The figure shows three views and two pictorial views of one solid part (mm, origin at its lowest corner). Answer the questions. Coordinates: 2 decimals unless noted, no trailing zeros. Order: outer loops, then holes, each group sorted by start corner. A loop starts at its lowest first (then second) coordinate and runs counter-clockwise, first axis right, second up.
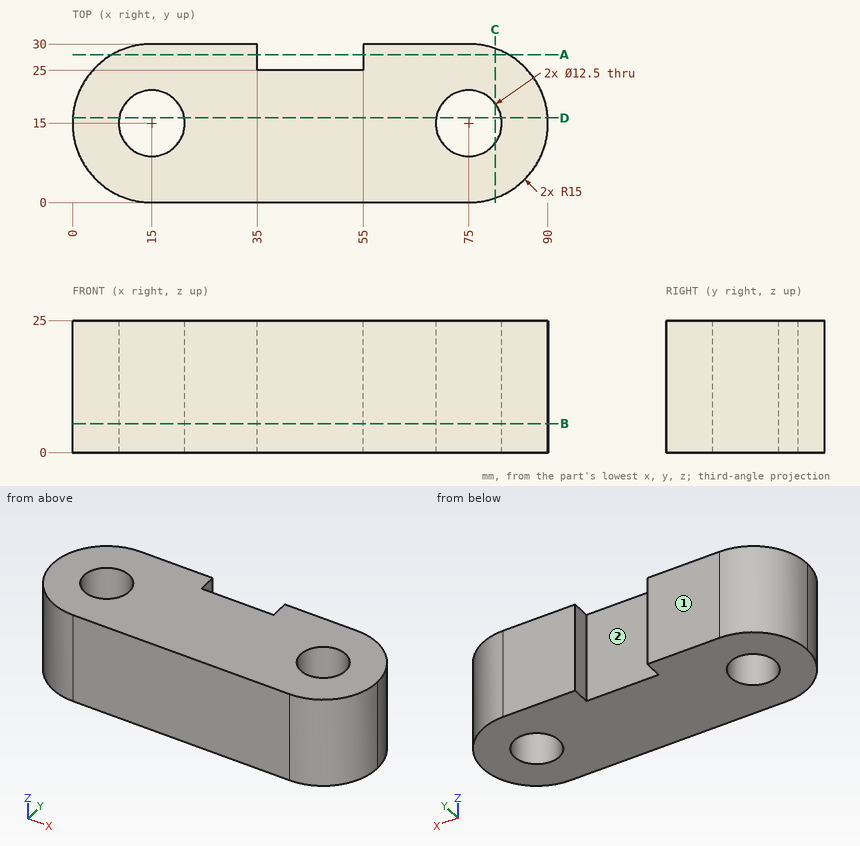
Q1. Determine the mould class of the marked faces 1 and 2 for opening direction X: +X half, -X half, draft (parallel to the pull), parting line (faces both ways), or undercut.
Q2. The part is cut by section B-B, the plane z = 5.5. Determine the outline of the cut face in (x, y).
Q3. The part is cut by section C-C, the plane x = 80. Determine the outline of the cut face in (y, z).
Q4. Each of these flat-tipped pins is pushed along its axis until it touches: P1, Ø11, axis at x = 75, y = 15, coming from the +Z side; P2, Ø3, axis at x = 44, y = 7.5, coming from the -Z side; P3, Ø5.5, axis at y = 28, z = 16.5, coming from the -X side; P4, Ø1.5, axis at y = 22, z = 16.5, coming from the -X side. Where does it stop, or does it pass through?
Q5. The part is cut by section A-A, the plane y = 28. Determine the outline of the cut face in (x, z).
Q6. The part is cut by section D-D, the plane y = 16. Determine the outline of the cut face in (x, z).
Q7. Straight lines are drawn through the part: L1, parallel to X at y = 16, z = 21.5; L2, parallel to X at y = 17, z = 24.25; L3, parallel to Y at x = 16.5, z = 23.5. For each, find the intervals that lie inside material, in ascending order.
Computed values:
1. face 1: draft
1. face 2: undercut
2. outline: (0, 15) arc R15 ccw to (15, 0) - (75, 0) arc R15 ccw to (90, 15) arc R15 ccw to (75, 30) - (55, 30) - (55, 25) - (35, 25) - (35, 30) - (15, 30) arc R15 ccw to start; hole circle Ø12.5 at (15, 15); hole circle Ø12.5 at (75, 15)
3. outline: (0.86, 0) - (11.25, 0) - (11.25, 25) - (0.86, 25) - close; (18.75, 0) - (29.14, 0) - (29.14, 25) - (18.75, 25) - close
4. P1: passes through
4. P2: stops at z = 0
4. P3: stops at x = 4.05
4. P4: stops at x = 1.36
5. outline: (7.52, 0) - (35, 0) - (35, 25) - (7.52, 25) - close; (55, 0) - (82.48, 0) - (82.48, 25) - (55, 25) - close
6. outline: (0.03, 0) - (8.83, 0) - (8.83, 25) - (0.03, 25) - close; (21.17, 0) - (68.83, 0) - (68.83, 25) - (21.17, 25) - close; (81.17, 0) - (89.97, 0) - (89.97, 25) - (81.17, 25) - close
7. L1: x = 0.03 to 8.83, 21.17 to 68.83, 81.17 to 89.97
7. L2: x = 0.13 to 9.08, 20.92 to 69.08, 80.92 to 89.87
7. L3: y = 0 to 8.93, 21.07 to 30
